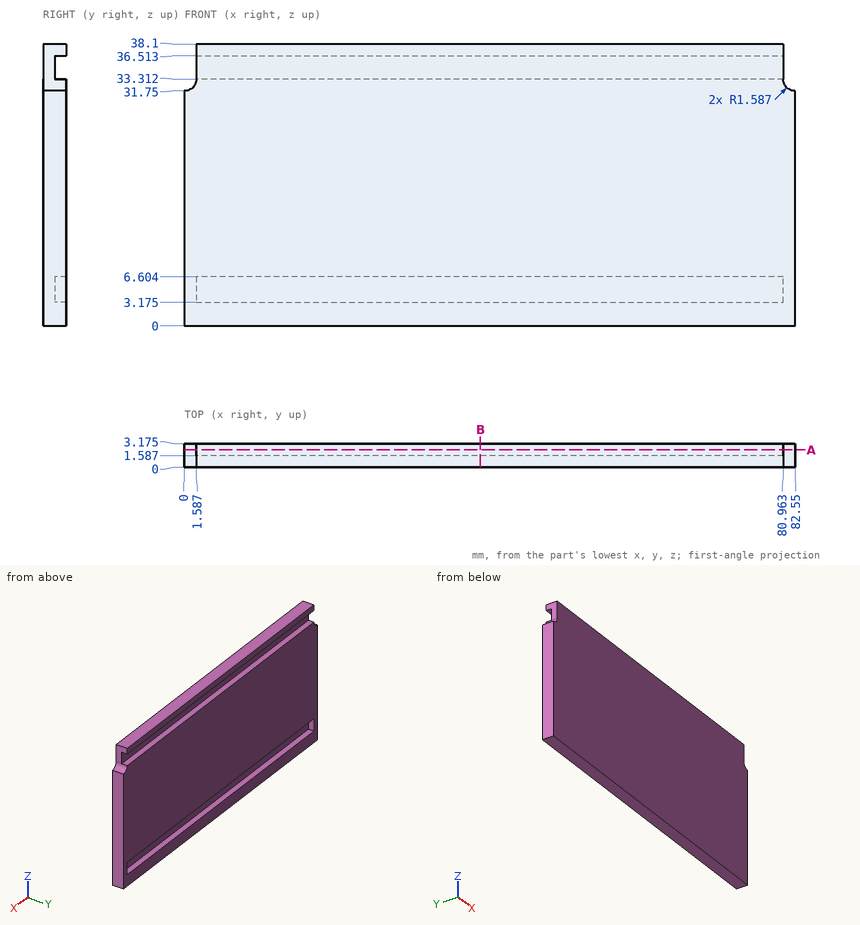
Verification items for this drawing (mm, ordinates from the low corner). Give positions to 0.01 mm unless a question says otherwise; leave off trailing zeros. Loops run counter-clockwise (first coordinate to the right, second up) from the corner with the lowest first, then second, coordinate; pieces in that order, holes last. Notation, with made-up numbers: M 63,-14 L 75,-14 A14 ccw 75,-3 Z; hole C -25.75,71.25 d4. An arc over 180 degrees is marked long. Answer as a JSON object with one key per item and string values. Group by question number.
Item 1: Sectioned sample at B-B on x = 40. Record the boundary of the cut face in (y, z) (1 decimal).
Item 2: Gauge pin test, flat ends, axial feed: pin 1 (2.5 mm diameter, centred on x = 57.5, z = 5.5, fed in from +Y) (1 decimal); pin 2 (2.5 mm diameter, centred on x = 39.5, z = 35, fed in from +Y). Record the tip position at first contact, or that the pin passes through.
Item 3: Material ranges on L1, parallel to Z at x = 3, y = 1.7 (1 decimal); L2, parallel to Y at x = 69, z = 33.5, recorded low to high.
Item 4: Sectioned sample at A-A on y = 2.35. Give the number of separate pieces and of enclosed holes in the cut face, plus the area to 3 significant figures.
Findings below:
{
 "1": {"outline": "M 0,0 L 3.2,0 L 3.2,3.2 L 1.6,3.2 L 1.6,6.6 L 3.2,6.6 L 3.2,33.3 L 1.6,33.3 L 1.6,36.5 L 3.2,36.5 L 3.2,38.1 L 0,38.1 Z"},
 "2": {"pin 1": "y = 3.2", "pin 2": "y = 1.59"},
 "3": {"L1": "0 to 3.2, 6.6 to 33.3, 36.5 to 38.1", "L2": "0 to 1.59"},
 "4": {"separate pieces": "2", "enclosed holes": "1", "area": "2,600 mm2"}
}
